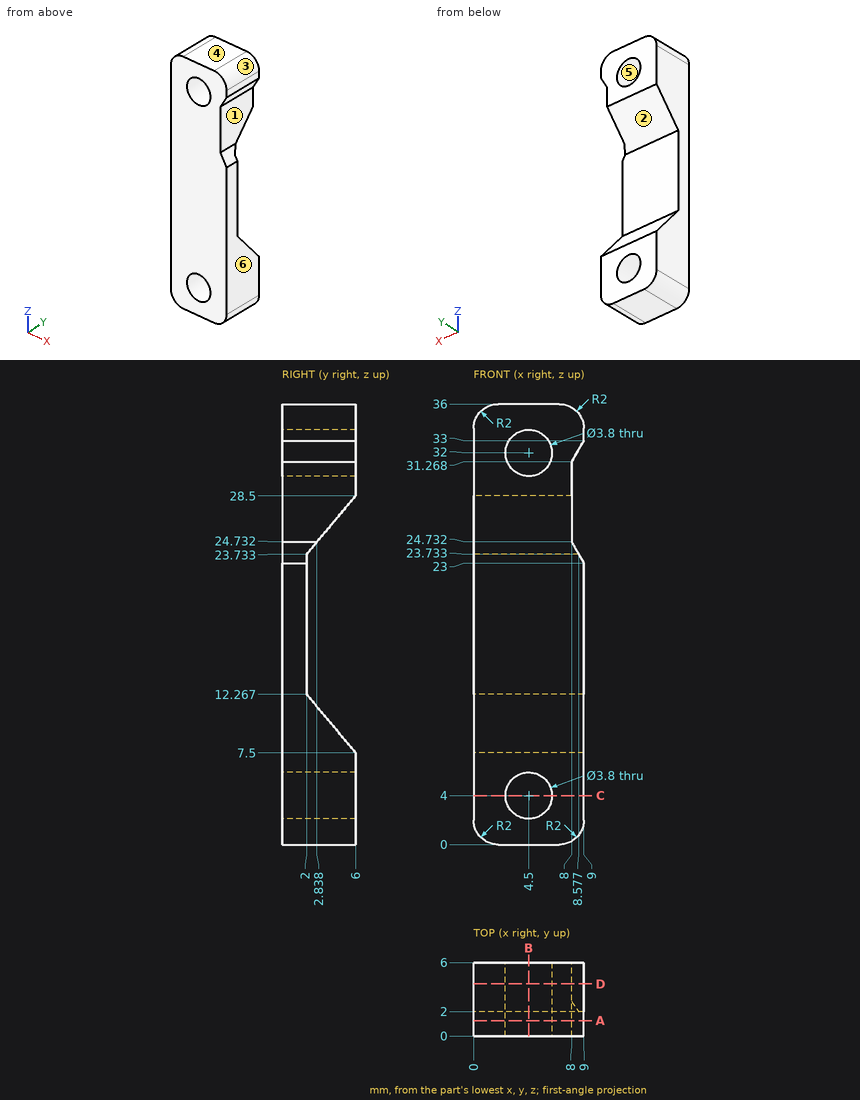
Design review of the part shown in the three views and the two pictorial views. Dimensions are in mm from the part's minimum x, y and z. A direction names the side the tool comes from. Coordinates: 2 decimals unless noted, no trailing zeros. Order: outer loops, then holes, each group sorted by start corner. A loop starts at its lowest first (then second) coordinate and runs counter-clockwise, first axis right, second up. Notation, with made-up numbers: (-7, 43.25) -> (-2, 43.25) arc R23 ccw to (-2, 64.25) -> close; hole circle Ø8 at (-25.75, -19.5). An arc over 180 degrees is marked (long way). Use one line per item in the form item = value. Start each with the question number.
(1) Add section C-C on z = 4. State the section outline as (x, y) points.
(2) Add section B-B on x = 4.5. State the section outline as (y, z) points.
(3) Insertion check: pin 1 (4.5 mm diameter, centred on x = 4.5, z = 4, fed in from -Y); pin 2 (2.5 mm diameter, centred on x = 6.5, z = 18, fed in from +Y); pin 3 (5 mm diameter, centred on x = 5, z = 22.5, fed in from +Y); pin 4 (2.5 mm diameter, centred on x = 4.5, z = 32, fed in from +Y). Each pin has a flat end and moves straight along its axis. Give the tip position at first contact, or say it passes through.
(4) The part is to be moulded in two halves that separate along Z. For the marked faces 4, 5 and 6, say which applies: +Z half, -Z half, draft (parallel to the pull), parting line (faces both ways), or undercut.
(5) For probe 1 along Z at (x, y) = (5.25, 4) (1 decimal); probe 2 along Z at (x, y) = (4.5, 2.95) (1 decimal); probe 3 along Z at (x, y) = (4, 1.75), list the stretches that pass through material, from the lowest coordinate up.
(6) Add section A-A on y = 1.25. State the section outline as (x, z) points, plus the area to 3 significant figures.
(7) For the marked faces 1, 2 and 3, list the 3-axis set-ups (+Z, -Z, +X, -X, +Y, -Y) from which the entire face can be reached by the end or side of a thin tool; tool diameter is ignored.
(8) Add section D-D on y = 4.25. State the section outline as (x, z) points (1 decimal).
Answer block:
q1.outline = (0, 0) -> (2.6, 0) -> (2.6, 6) -> (0, 6) -> close; (6.4, 0) -> (9, 0) -> (9, 6) -> (6.4, 6) -> close
q2.outline = (0, 0) -> (6, 0) -> (6, 2.1) -> (0, 2.1) -> close; (0, 5.9) -> (6, 5.9) -> (6, 7.5) -> (2, 12.27) -> (2, 23.73) -> (6, 28.5) -> (6, 30.1) -> (0, 30.1) -> close; (0, 33.9) -> (6, 33.9) -> (6, 36) -> (0, 36) -> close
q3.pin_1 = 0
q3.pin_2 = 2
q3.pin_3 = 3.06
q3.pin_4 = through
q4.face_4 = +Z half
q4.face_5 = undercut
q4.face_6 = draft
q5.probe_1 = 0 to 2.3, 5.7 to 9.9, 26.1 to 30.3, 33.7 to 36
q5.probe_2 = 0 to 2.1, 5.9 to 11.1, 24.9 to 30.1, 33.9 to 36
q5.probe_3 = 0 to 2.17, 5.83 to 30.17, 33.83 to 36
q6.outline = (0, 2) arc R2 ccw to (2, 0) -> (7, 0) arc R2 ccw to (9, 2) -> (9, 23) -> (8, 24.73) -> (8, 31.27) -> (9, 33) -> (9, 34) arc R2 ccw to (7, 36) -> (2, 36) arc R2 ccw to (0, 34) -> close; hole circle Ø3.8 at (4.5, 4); hole circle Ø3.8 at (4.5, 32)
q6.area = 290 mm²
q7.face_1 = +X, +Y, -Y
q7.face_2 = +X, -X, +Y
q7.face_3 = +Z, +X, +Y, -Y
q8.outline = (0, 2) arc R2 ccw to (2, 0) -> (7, 0) arc R2 ccw to (9, 2) -> (9, 9.6) -> (0, 9.6) -> close; (0, 26.4) -> (8, 26.4) -> (8, 31.3) -> (9, 33) -> (9, 34) arc R2 ccw to (7, 36) -> (2, 36) arc R2 ccw to (0, 34) -> close; hole circle Ø3.8 at (4.5, 4); hole circle Ø3.8 at (4.5, 32)
